```python
from build123d import *

# Parameters (mm, degrees)
SKETCH1_R           = 25.4
BOSS_EXTRUDE1_DEPTH = 3.175
SKETCH2_R           = 1.7272
CUT_EXTRUDE1_DEPTH  = 4.175
SKETCH3_R           = 3.2004
CUT_EXTRUDE2_DEPTH  = 4.175
SKETCH4_R           = 1.499997
CUT_EXTRUDE3_DEPTH  = 4.175


with BuildPart() as part:
    # Sketch1 → Boss-Extrude1 (new body)
    with BuildSketch(Plane(origin=(0, 0, 0), x_dir=(1, 0, 0), z_dir=(0, 1, 0))):
        Circle(SKETCH1_R)
    extrude(amount=BOSS_EXTRUDE1_DEPTH)

    # Sketch2 → Cut-Extrude1 (cut, through all)
    with BuildSketch(Plane(origin=(0, 3.175, 0), x_dir=(1, 0, 0), z_dir=(0, 1, 0))):
        with Locations((-22.14499, 0)):
            Circle(SKETCH2_R)
    extrude(amount=-CUT_EXTRUDE1_DEPTH, mode=Mode.SUBTRACT)

    # Sketch3 → Cut-Extrude2 (cut, through all)
    with BuildSketch(Plane(origin=(0, 3.175, 0), x_dir=(1, 0, 0), z_dir=(0, 1, 0))):
        Circle(SKETCH3_R)
    extrude(amount=-CUT_EXTRUDE2_DEPTH, mode=Mode.SUBTRACT)

    # Sketch4 → Cut-Extrude3 (cut, through all)
    with BuildSketch(Plane(origin=(0, 3.175, 0), x_dir=(1, 0, 0), z_dir=(0, 1, 0))):
        with Locations((0, 7.999984)):
            Circle(SKETCH4_R)
        with Locations((0, -7.999984)):
            Circle(SKETCH4_R)
        with Locations((7.999984, 0)):
            Circle(SKETCH4_R)
    extrude(amount=-CUT_EXTRUDE3_DEPTH, mode=Mode.SUBTRACT)


solid = part.part
```
Geometry: final body of the model. Coordinates: model frame, mm. Round coordinates to 2 decimals unless told otherwise and drop trailing zeros. Order: outer loops, then holes, each group sorted by start corner. A loop starts at its lowest first (then second) coordinate and runs counter-clockwise, first axis right, second up. Notation, with made-up numbers: M 26,50.5 L 72,50.5 A11 ccw 72,67.5 Z; hole C -14,39.25 d5. An arc over 180 degrees is marked long. Use one line per item in the form item = value. Start each with the question number.
Q1. Cut plane D-D (z = -18.5). Return loops of the section in (x, y) (3 decimals), and give its area (3 significant figures).
Q2. Cut plane C-C (y = 1.35). Return loops of the section in (x, z).
Q3. Material intervals for line 1 (Z direction, x = 0, y = 1.4); line 2 (X direction, y = 1.2, z = 0); line 3 (Z direction, x = -1, y = 0.8), sorted ascending. Write a range as [from, to].
Q4. Pin query (flat end, axial travel): pin 1 Ø1.5 at (y, z) = (3, -3) entering from +X; pin 2 Ø1.5 at (x, y) = (-2.5, 1.5) entering from +Z. Return the tip coordinate at first contact, or that it passes through.
Q5. Cut plane B-B (z = 0). Return loops of the section in (x, y) (3 decimals).
Q6. Cut plane A-A (x = 0). Return loops of the section in (y, z) (3 decimals).
Q7. Mould query, pull axis Z, two halves, no side actions, for faces 1 (the face through (-5.506, 1.565, 24.796)), 2 (the face through (-0.195, 1.61, -9.487)), 3 (the face through (5, 0, 0)). Classes: +Z half, -Z half, draft (parallel to the pull), parting line (faces both ways), or undercut.
Geometry results:
q1.outline = M -17.404,0 L 17.404,0 L 17.404,3.175 L -17.404,3.175 Z
q1.area = 111 mm^2
q2.outline = C 0,0 d50.8; hole C -22.14,0 d3.45; hole C 0,0 d6.4; hole C 0,-8 d3; hole C 0,8 d3; hole C 8,0 d3
q3.line_1 = [-25.4, -9.5], [-6.5, -3.2], [3.2, 6.5], [9.5, 25.4]
q3.line_2 = [-25.4, -23.87], [-20.42, -3.2], [3.2, 6.5], [9.5, 25.4]
q3.line_3 = [-25.38, -9.12], [-6.88, -3.04], [3.04, 6.88], [9.12, 25.38]
q4.pin_1 = 25.3
q4.pin_2 = 25.34
q5.outline = M -25.4,0 L -23.872,0 L -23.872,3.175 L -25.4,3.175 Z; M -20.418,0 L -3.2,0 L -3.2,3.175 L -20.418,3.175 Z; M 3.2,0 L 6.5,0 L 6.5,3.175 L 3.2,3.175 Z; M 9.5,0 L 25.4,0 L 25.4,3.175 L 9.5,3.175 Z
q6.outline = M 0,-25.4 L 3.175,-25.4 L 3.175,-9.5 L 0,-9.5 Z; M 0,-6.5 L 3.175,-6.5 L 3.175,-3.2 L 0,-3.2 Z; M 0,3.2 L 3.175,3.2 L 3.175,6.5 L 0,6.5 Z; M 0,9.5 L 3.175,9.5 L 3.175,25.4 L 0,25.4 Z
q7.face_1 = parting line
q7.face_2 = undercut
q7.face_3 = draft
